from build123d import *

# Parameters (mm, degrees)
F1_DEPTH = 31.75
F0_W     = 31.75
F0_H     = 31.75
F2_DEPTH = 92.075
F0_H_2   = 88.9
F3_DEPTH = 73.025
F4_DEPTH = 53.975
F5_DEPTH = 53.975
F6_DEPTH = 92.075
F7_DEPTH = 73.025
F8_DEPTH = 31.75


with BuildPart() as f1:
    # F0 (on Top) → F1 (new body)
    with BuildSketch(Plane.XY):
        Polygon((-57.15, 0), (0, 0), (0, 50.8), (-15.875, 50.8), (-15.875, 101.6), (0, 101.6), (0, 152.4), (-57.15, 152.4), (-57.15, 120.65), (-57.15, 31.75), align=None)
    extrude(amount=F1_DEPTH)

    # F0 (on Top) → F2 (join)
    with BuildSketch(Plane.XY):
        with Locations((-73.025, 136.525)):
            Rectangle(F0_W, F0_H)
        with Locations((-73.025, 15.875)):
            Rectangle(F0_W, F0_H)
    extrude(amount=F2_DEPTH)

    # F0 (on Top) → F3 (join)
    with BuildSketch(Plane.XY):
        with Locations((-73.025, 76.2)):
            Rectangle(F0_W, F0_H_2)
    extrude(amount=F3_DEPTH)

    # F0 (on Top) → F4 (join)
    with BuildSketch(Plane.XY):
        with BuildLine():
            Line((-127, 0), (-88.9, 0))
            Line((-88.9, 0), (-88.9, 31.75))
            Line((-88.9, 31.75), (-88.9, 120.65))
            Line((-88.9, 120.65), (-88.9, 152.4))
            Line((-88.9, 152.4), (-127, 152.4))
            Line((-127, 152.4), (-127, 92.075))
            ThreePointArc((-127, 92.075), (-115.7746798487, 87.4253201513), (-111.125, 76.2))
            ThreePointArc((-111.125, 76.2), (-115.7746798487, 64.9746798487), (-127, 60.325))
            Line((-127, 60.325), (-127, 0))
        make_face()
    extrude(amount=F4_DEPTH)

    # F0 (on Top) → F5 (join)
    with BuildSketch(Plane.XY):
        with BuildLine():
            Line((-165.1, 0), (-127, 0))
            Line((-127, 0), (-127, 60.325))
            ThreePointArc((-127, 60.325), (-142.875, 76.2), (-127, 92.075))
            Line((-127, 92.075), (-127, 152.4))
            Line((-127, 152.4), (-165.1, 152.4))
            Line((-165.1, 152.4), (-165.1, 120.65))
            Line((-165.1, 120.65), (-165.1, 31.75))
            Line((-165.1, 31.75), (-165.1, 0))
        make_face()
    extrude(amount=F5_DEPTH)

    # F0 (on Top) → F6 (join)
    with BuildSketch(Plane.XY):
        with Locations((-180.975, 136.525)):
            Rectangle(F0_W, F0_H)
        with Locations((-180.975, 15.875)):
            Rectangle(F0_W, F0_H)
    extrude(amount=F6_DEPTH)

    # F0 (on Top) → F7 (join)
    with BuildSketch(Plane.XY):
        with Locations((-180.975, 76.2)):
            Rectangle(F0_W, F0_H_2)
    extrude(amount=F7_DEPTH)

    # F0 (on Top) → F8 (join)
    with BuildSketch(Plane.XY):
        Polygon((-254, 0), (-196.85, 0), (-196.85, 31.75), (-196.85, 120.65), (-196.85, 152.4), (-254, 152.4), (-254, 101.6), (-238.125, 101.6), (-238.125, 50.8), (-254, 50.8), align=None)
    extrude(amount=F8_DEPTH)


solid = f1.part
The listing builds one solid part. Answer for the finished solid, in the listing's coordinates (mm). A direction names the side the tool comes from. Coordinates: 2 decimals unless noted, no trailing zeros. Loops run counter-clockwise (first coordinate to the right, second up) from the corner with the lowest first, then second, coordinate; pieces in that order, holes last. Notation, with made-up numbers: (60.5, 61.25) -> (72.5, 61.25) arc R23 ccw to (72.5, 83.25) -> close; hole circle Ø5 at (29, 30). An arc over 180 degrees is marked (long way). Write item = value, one per line. Start each with the question number.
1) The mould has two halves that part along X. Classify faces 6 (the face through (-88.9, 75, 69)), 7 (the face through (-15.875, 76, 16)), 8 (the face through (-129, 0, 35)), 9 (the face through (-165.1, 75, 69)): released by +X, released by -X, zero draft, split by the parting line, or undercut.
2) A cutting plane is placed at D-D (x = -184). Give the vertices of the cut face in (y, z) (3 decimals).
3) Given pin 1 Ø6 at (y, z) = (69.5, 72.5) entering from +X; pin 2 Ø12 at (y, z) = (130.5, 79.5) entering from -X; pin 3 Ø17 at (x, y) = (-229.5, 53) entering from +Z; pin 4 Ø1 at (x, z) = (-56, 54.5) entering from +Y, each flat-ended and moving along its own axis, determine where each tip first touches the part or whether it passes through.
4) A tool of negligible diameter and unlimited length cuts with its end or side. For faces 1 (the face through (-181, 137, 92.075)), 2 (the face through (-8, 101.6, 16)), 3 (the face through (-181, 120.65, 82)), 4 (the face through (-29, 77, 31.75)), 5 (the face through (-246, 50.8, 16)), from which of +Z, -Z, +X, -X, +Y, -Y can it reach the whole face along a straight path? Write none if from no direction.
5) Straight lines are drawn through the part: line 1 (X direction, y = 8, z = 54.5); line 2 (Z direction, x = -198, y = 43.5); line 3 (Z direction, x = -176, y = 72) (3 decimals). For each, find the intervals that lie inside material, in ascending order. Write a range as from..to.
6) A cutting plane is placed at B-B (y = 112.5). Give the vertices of the cut face in (x, z) (3 decimals).
7) A cutting plane is placed at A-A (z = 14.5). Give the vertices of the cut face in (x, y) (3 decimals), then the cut area to 3 significant figures.
8) A cutting plane is placed at C-C (z = 76). Give the vertices of the cut face in (x, y), then the cut area to 3 significant figures.
Responses:
q1.face_6 = undercut
q1.face_7 = released by +X
q1.face_8 = zero draft
q1.face_9 = undercut
q2.outline = (0, 0) -> (152.4, 0) -> (152.4, 92.075) -> (120.65, 92.075) -> (120.65, 73.025) -> (31.75, 73.025) -> (31.75, 92.075) -> (0, 92.075) -> close
q3.pin_1 = -57.15
q3.pin_2 = -196.85
q3.pin_3 = 31.75
q3.pin_4 = through
q4.face_1 = +Z, +X, -X, +Y, -Y
q4.face_2 = +Z, -Z, +X
q4.face_3 = +Z, +X, -X
q4.face_4 = +Z, +X, +Y, -Y
q4.face_5 = +Z, -Z, -X
q5.line_1 = -196.85..-165.1, -88.9..-57.15
q5.line_2 = 0..31.75
q5.line_3 = 0..73.025
q6.outline = (-254, 0) -> (0, 0) -> (0, 31.75) -> (-57.15, 31.75) -> (-57.15, 73.025) -> (-88.9, 73.025) -> (-88.9, 53.975) -> (-165.1, 53.975) -> (-165.1, 73.025) -> (-196.85, 73.025) -> (-196.85, 31.75) -> (-254, 31.75) -> close
q7.outline = (-254, 0) -> (0, 0) -> (0, 50.8) -> (-15.875, 50.8) -> (-15.875, 101.6) -> (0, 101.6) -> (0, 152.4) -> (-254, 152.4) -> (-254, 101.6) -> (-238.125, 101.6) -> (-238.125, 50.8) -> (-254, 50.8) -> close; hole circle Ø31.75 at (-127, 76.2)
q7.area = 36,300 mm²
q8.outline = (-196.85, 0) -> (-165.1, 0) -> (-165.1, 31.75) -> (-196.85, 31.75) -> close; (-196.85, 120.65) -> (-165.1, 120.65) -> (-165.1, 152.4) -> (-196.85, 152.4) -> close; (-88.9, 0) -> (-57.15, 0) -> (-57.15, 31.75) -> (-88.9, 31.75) -> close; (-88.9, 120.65) -> (-57.15, 120.65) -> (-57.15, 152.4) -> (-88.9, 152.4) -> close
q8.area = 4,030 mm²
